from build123d import *

# Parameters (mm, degrees)
SKETCH_W         = 142
SKETCH_H         = 124
PAD_DEPTH        = 4
HOLE_D           = 3.4
HOLE_DEPTH       = 25
HOLE_CSINK_D     = 6.1
HOLE_CSINK_ANGLE = 90


with BuildPart() as part:
    # Sketch → Pad (new body)
    with BuildSketch(Plane.XY):
        Rectangle(SKETCH_W, SKETCH_H)
    extrude(amount=PAD_DEPTH)

    # Hole
    with Locations(Plane(origin=(0, 0, 0), x_dir=(1, 0, 0), z_dir=(0, 0, -1))):
        with Locations((-68, 59), (-68, -59), (68, -59), (68, 59)):
            CounterSinkHole(HOLE_D / 2, HOLE_CSINK_D / 2, depth=HOLE_DEPTH, counter_sink_angle=HOLE_CSINK_ANGLE)


solid = part.part
Verification items for the finished model (mm, model axes). Coordinates: 2 decimals unless noted, no trailing zeros. Use CSV: the item, a comma, the result in double quotes.
Q1. Go/stop test with flat-tipped pins: P1, Ø5.5, axis at x = 68, y = 59, coming from the +Z side; P2, Ø5.5, axis at x = -68, y = -59, coming from the -Z side; P3, Ø2.5, axis at x = 68, y = -59, coming from the -Z side. Record where each tip stops, or that it passes through.
Computed values:
P1,"z = 4"
P2,"z = 0.3"
P3,"through"
Q2. Mould release check, pull along X, two halves, no side actions. Record for faces 1 (the cylindrical face through (69.7, 58.93, 2.69)), 2 (the flat face through (-71, -1, 2)), 3 (the flat face through (-1, 1, 0)): pulls with the +X half, pulls with the -X half, needs draft (parallel to the pull), parting line crosses it, or undercut.
Computed values:
face 1,"undercut"
face 2,"pulls with the -X half"
face 3,"needs draft"
Q3. Thickness scan on line 1 along X through (y, z) = (59, 3.4); line 2 along Y through (x, z) = (-68, 3). Record the ranges inside material, lowest first. Write a range as [from, to].
Computed values:
line 1,"[-71, -69.7], [-66.3, 66.3], [69.7, 71]"
line 2,"[-62, -60.7], [-57.3, 57.3], [60.7, 62]"
